Could you check a few things on this model? Use its own coordinates, in mm. Face numbers are marked on the shaded views. A direction names the side the tool comes from. Give positions to 0.01 mm unless a question says otherwise; leave off trailing zeros. Order: outer loops, then holes, each group sorted by start corner. A loop starts at its lowest first (then second) coordinate and runs counter-clockwise, first axis right, second up. Notation, with made-up numbers: M -5,30.5 L 38,30.5 A26 ccw 38,59.5 Z; hole C 35,-2.75 d6. An arc over 180 degrees is marked long. Use a Markdown table: item, result. Add a question column.
Item 1: Suppose I cut it at A-A on y = 46. Write out the boundary of the cut face in (x, z), plus the area to 3 significant figures.
Item 2: Suppose I cut it at D-D on x = 101.5. Write out the boundary of the cut face in (y, z), plus the area to 3 significant figures.
Item 3: Suppose I cut it at C-C on z = 12. Write out the boundary of the cut face in (x, y).
Item 4: I'm going to push flat-ended pins straight in: pin 1 Ø1 at (x, z) = (-28.5, 15) entering from +Y; pin 2 Ø0.6 at (x, z) = (245.5, 1.5) entering from +Y; pin 3 Ø3 at (x, z) = (349, 2) entering from -Y. Where does each tip first touch, or does it pass through?
Item 5: Suppose I cut it at B-B on x = 0. Write out the boundary of the cut face in (y, z), plus the area to 3 significant figures.
Item 6: If I drill on L1, parallel to Y at x = -416, z = 15; L2, parallel to Y at x = 227, z = 3.25, over which ranges is the centre line in solid material (lowest first)? Write a range as from..to.
Item 7: For the marked faces 1 and 2, which set-ups out of +Z, -Z, +X, -X, +Y, -Y let a thin tool reach every point of the face, with its end or its side?
Autodesk Inventor part; units mm, degrees
ref_plane "YZ Plane" through (0, 0, 0) normal (1, 0, 0) x (0, 1, 0)
ref_plane "XZ Plane" through (0, 0, 0) normal (0, 1, 0) x (-1, 0, 0)
ref_plane "XY Plane" through (0, 0, 0) normal (0, 0, 1) x (1, 0, 0)
sketch "Sketch1" plane through (0, 0, 0) normal (0, 0, 1) x (1, 0, 0)
  line L0 (-490, 68) -> (490, 68)
  line L1 (490, 68) -> (490, 0)
  line L2 (490, 0) -> (-490, 0)
  line L3 (-490, 0) -> (-490, 68)
  point P0 (0, 0)
  point P1 (0, 0)
  dimension "d0" = 980
  dimension "d1" = 68
extrude "Plate1" add sketch "Sketch1" along normal blind 2
sketch "Sketch2" plane through (490, 2, 0) normal (0, -1, 0) x (1, 0, 0)
  line L0 (-980, 0) -> (0, 0)
  line L1 (0, 0) -> (0, 20)
  line L2 (0, 20) -> (-980, 20)
  line L3 (-980, 20) -> (-980, 0)
edge flange "Flange1" height 20 angle 90 thickness 2 bend radius 2.75 thickness toward (0, -1, 0) relief round relief width 2 relief depth 1 edges at (0, 0, 2) wall of the first edge with corners at (-490, 2, 0) (490, 2, 0) (490, 2, 20) (-490, 2, 20)
bend "Bend1"
corner "Corner1"
sketch "Sketch5" plane through (0, 0, 0) normal (0, 0, -1) x (-1, 0, 0)
  line L0 (490, 68) -> (-490, 68)
  line L1 (490, 0) -> (-490, 0)
  circle A0 centre (0, 68) radius 35
  line L2 (243.95, 68) -> (246.05, 68)
  line L3 (246.05, 68) -> (246.05, 29)
  line L4 (246.05, 29) -> (243.95, 29)
  line L5 (243.95, 29) -> (243.95, 68)
  line L6 (-243.95, 68) -> (-246.05, 68)
  line L7 (-246.05, 68) -> (-246.05, 29)
  line L8 (-246.05, 29) -> (-243.95, 29)
  line L9 (-243.95, 29) -> (-243.95, 68)
  line L10 (0, 68) -> (0, 0) construction
  point P0 (0, 0)
  point P1 (245, 29)
  point P2 (-245, 29)
  point P3 (-35, 68)
  point P4 (35, 68)
  dimension "d45" = 70
  dimension "d48" = 2.1
  dimension "d49" = 490
  dimension "d51" = 29
  dimension "d52" = 39
extrude "Extrusion1" cut sketch "Sketch5" against normal through all contours L3 L4 L5 L0 | L9 L8 L7 L0 | A0 L0 picked at (-5.3545, 54.8926)
sketch "Sketch9" plane through (0, 0, 2) normal (0, 0, 1) x (1, 0, 0)
  line L0 (485.6141, 29.596) -> (485.6141, 17.596) construction
  line L1 (485.6141, 17.596) -> (285.6141, 17.596) construction
  line L2 (285.6141, 17.596) -> (285.6141, 29.596) construction
  line L3 (285.6141, 29.596) -> (485.6141, 29.596) construction
  line L4 (-490, 68) -> (490, 68)
  point P0 (0, 0)
  point P1 (1.05, 68)
  dimension "d40" = 200
  dimension "d41" = 12
mark "Mark2"
equation "\"d1\" = СПИНА_Стрингер_2_высота"
equation "\"d2\" = Thickness"
equation "\"d3\" = BendReliefWidth"
equation "\"d4\" = BendReliefDepth"
equation "\"d5\" = MinimumRemnant"
equation "\"d6\" = TransitionRadius"
equation "\"d9\" = BendRadius"
equation "\"d10\" = CornerReliefSize"
equation "\"d11\" = GapSize"
equation "\"d12\" = JacobiRadiusSize"
equation "\"BendReliefWidth\" = Thickness"
equation "\"BendReliefDepth\" = 0.5 * Thickness"
equation "\"CornerReliefSize\" = 4 * Thickness"
equation "\"MinimumRemnant\" = 2 * Thickness"
equation "\"TransitionRadius\" = BendRadius"
equation "\"JacobiRadiusSize\" = BendRadius"
equation "\"GapSize\" = Thickness"
properties part number "MSC 062 stringer back ^^" material "Stainless Steel"
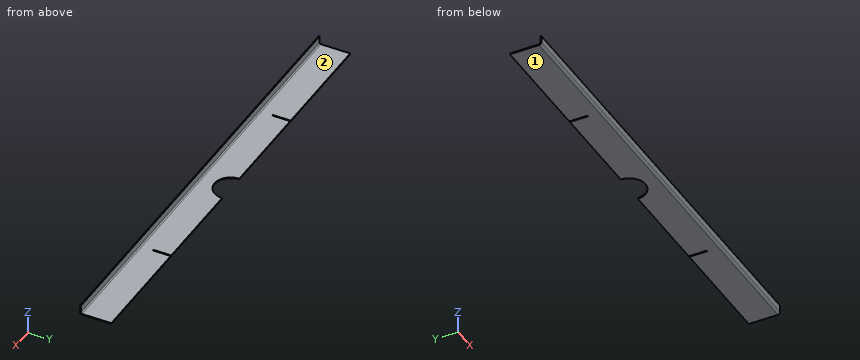
Findings below:
| question | item | result |
|---|---|---|
| 1 | outline | M -490,0 L -246.05,0 L -246.05,2 L -490,2 Z; M -243.95,0 L -27.22,0 L -27.22,2 L -243.95,2 Z; M 27.22,0 L 243.95,0 L 243.95,2 L 27.22,2 Z; M 246.05,0 L 490,0 L 490,2 L 246.05,2 Z |
| 1 | area | 1,840 mm^2 |
| 2 | outline | M 0,4.75 A4.75 ccw 4.75,0 L 68,0 L 68,2 L 4.75,2 A2.75 cw 2,4.75 L 2,20 L 0,20 Z |
| 2 | area | 169 mm^2 |
| 3 | outline | M -490,0 L 490,0 L 490,2 L -490,2 Z |
| 4 | pin 1 | stops at y = 2 |
| 4 | pin 2 | stops at y = 29 |
| 4 | pin 3 | stops at y = 0.17 |
| 5 | outline | M 0,4.75 A4.75 ccw 4.75,0 L 33,0 L 33,2 L 4.75,2 A2.75 cw 2,4.75 L 2,20 L 0,20 Z |
| 5 | area | 98.8 mm^2 |
| 6 | L1 | y = 0..2 |
| 6 | L2 | y = 0.24..2.45 |
| 7 | face 1 | -Z, +X, -X, +Y, -Y |
| 7 | face 2 | +Z, +X, -X, +Y |
